```python
from build123d import *

# Parameters (mm, degrees)
F5_D = 5
F6_R = 3
F8_D = 5


with BuildPart() as f1:
    # F0 (on Front) → F1 (revolve)
    with BuildSketch(Plane.XZ):
        Polygon((-36.025, 0), (-26.025, 0), (-26.025, 20), (-19, 20), (-19, 40), (-66, 40), (-66, 30), (-36.025, 30), align=None)
    revolve(axis=Axis((0, 0, -7.200188), (0, 0, -1)))

    # F5 (through all)
    with Locations(Plane.XY.offset(40)):
        with Locations((0, 51.0125), (0, -51.0125)):
            Hole(F5_D / 2)

    # F6
    f6_edges = [f1.edges().sort_by_distance(p)[0] for p in [
        (26.025, 0, 0),
    ]]
    fillet(f6_edges, radius=F6_R)

    # F8 (through all)
    with Locations(Plane.XY.offset(40)):
        with Locations((51.0125, 0), (-51.153772, 0)):
            Hole(F8_D / 2)


solid = f1.part
```
Geometry check sheet. Reference: the model listing, model coordinates, mm. A direction names the side the tool comes from. Round coordinates to 2 decimals unless told otherwise and drop trailing zeros. Write each loop counter-clockwise with the first axis right and the second up, starting at its lowest first coordinate (ties: lowest second). Pieces come first, ordered by that corner, then holes. Notation, with made-up numbers: (89, 71.5) -> (119, 71.5) arc R19 ccw to (119, 96.5) -> close; hole circle Ø11 at (-18, -11). An arc over 180 degrees is marked (long way). Put each result on its own line as item: value.
1) Cross-section at A-A, the plane y = 0. Enter the section's corners in (x, z) (1 decimal).
Recorded:
outline: (-66, 30) -> (-53.7, 30) -> (-53.7, 40) -> (-66, 40) -> close; (-48.7, 30) -> (-36, 30) -> (-36, 0) -> (-29, 0) arc R3 ccw to (-26, 3) -> (-26, 20) -> (-19, 20) -> (-19, 40) -> (-48.7, 40) -> close; (19, 20) -> (26, 20) -> (26, 3) arc R3 ccw to (29, 0) -> (36, 0) -> (36, 30) -> (48.5, 30) -> (48.5, 40) -> (19, 40) -> close; (53.5, 30) -> (66, 30) -> (66, 40) -> (53.5, 40) -> close
2) Cross-section at D-D, the plane z = 36.5. Enter the section's corners in (x, y).
Recorded:
outline: circle Ø132 at (0, 0); hole circle Ø5 at (-51.15, 0); hole circle Ø38 at (0, 0); hole circle Ø5 at (0, -51.01); hole circle Ø5 at (0, 51.01); hole circle Ø5 at (51.01, 0)
3) Depth check by flat-ended pin: P1, Ø3, axis at x = 0, y = -51.01, coming from the -Z side; P2, Ø12, axis at y = 50.5, z = 33, coming from the +X side; P3, Ø6.5, axis at x = -51.15, y = 0, coming from the -Z side; P4, Ø8, axis at x = -9.5, z = 33.5, coming from the +Y side. Enter the tip coordinate at first touch or a pass-through.
Recorded:
P1: passes through
P2: stops at x = 48.74
P3: stops at z = 30
P4: stops at y = 65.77
4) Thickness scan on probe 1 along Y at (x, z) = (0, 33.25); probe 2 along Z at (x, y) = (-40, 32); probe 3 along Y at (x, z) = (9, 26). Record the ranges inside material, lowest first. Write a range as from..to.
Recorded:
probe 1: y = -66..-53.51, -48.51..-19, 19..48.51, 53.51..66
probe 2: z = 30..40
probe 3: y = -34.88..-16.73, 16.73..34.88
5) Access from +Z, -Z, +X, -X, +Y, -Y to the whole of each face (thin tool, end or side, straight path). Record for faces 4 (the face through (-1.8, -19.2, 20)), 5 (the face through (-1.34, -48.9, 34.93)).
Recorded:
face 4: -Z
face 5: +Z, -Z
6) Cross-section at C-C, the plane z = 11. Enter the section's corners in (x, y) (3 decimals), plus the area to 3 significant figures.
Recorded:
outline: circle Ø72.05 at (0, 0); hole circle Ø52.05 at (0, 0)
area: 1,950 mm2
7) Cross-section at B-B, the plane x = 0. Enter the section's corners in (y, z) (1 decimal).
Recorded:
outline: (-66, 30) -> (-53.5, 30) -> (-53.5, 40) -> (-66, 40) -> close; (-48.5, 30) -> (-36, 30) -> (-36, 0) -> (-29, 0) arc R3 ccw to (-26, 3) -> (-26, 20) -> (-19, 20) -> (-19, 40) -> (-48.5, 40) -> close; (19, 20) -> (26, 20) -> (26, 3) arc R3 ccw to (29, 0) -> (36, 0) -> (36, 30) -> (48.5, 30) -> (48.5, 40) -> (19, 40) -> close; (53.5, 30) -> (66, 30) -> (66, 40) -> (53.5, 40) -> close
8) Release check for a two-part mould opening along Y. For faces 1 (the face through (-1.344, 53.121, 34.93)), 2 (the face through (7.81, -35.17, 14.79)), 3 (the face through (-3, 30, 0)) record: pulls with the +Y half, pulls with the -Y half, needs draft (parallel to the pull), parting line crosses it, or undercut.
Recorded:
face 1: undercut
face 2: parting line crosses it
face 3: needs draft
